```python
from build123d import *

# Parameters (mm, degrees)
F1_DEPTH = 5


with BuildPart() as f1:
    # F0 (on Top) → F1 (new body)
    with BuildSketch(Plane.XY):
        with BuildLine():
            ThreePointArc((-2.891459, -1.483901), (0, 3.25), (2.891459, -1.483901))
            ThreePointArc((2.891459, -1.483901), (2.566364, -2.666148), (2.741421, -3.879717))
            Line((2.741421, -3.879717), (4.605052, -9))
            Line((4.605052, -9), (25, -9))
            Line((25, -9), (25, 2))
            ThreePointArc((25, 2), (23, 4), (25, 6))
            Line((25, 6), (25, 7))
            ThreePointArc((25, 7), (24.707107, 7.707107), (24, 8))
            Line((24, 8), (-24, 8))
            ThreePointArc((-24, 8), (-24.707107, 7.707107), (-25, 7))
            Line((-25, 7), (-25, 6))
            ThreePointArc((-25, 6), (-23, 4), (-25, 2))
            Line((-25, 2), (-25, -9))
            Line((-25, -9), (-4.605052, -9))
            Line((-4.605052, -9), (-2.741421, -3.879717))
            ThreePointArc((-2.741421, -3.879717), (-2.566364, -2.666148), (-2.891459, -1.483901))
        make_face()
    extrude(amount=F1_DEPTH)


solid = f1.part
```
Design review of the part built by this model. Coordinates are the model's own, in mm. A direction names the side the tool comes from. Coordinates: 2 decimals unless noted, no trailing zeros. Order: outer loops, then holes, each group sorted by start corner. A loop starts at its lowest first (then second) coordinate and runs counter-clockwise, first axis right, second up. Notation, with made-up numbers: (60, 14.5) - (75, 14.5) arc R20 cw to (75, 41.5) - close; hole circle Ø6 at (35, -29.75). An arc over 180 degrees is marked (long way). Answer in a Markdown table with one row per item.
(1) Consider section A-A on y = 0. State the section outline as (x, z) points.
Checked values:
| item | result |
|---|---|
| outline | (-25, 0) - (-3.25, 0) - (-3.25, 5) - (-25, 5) - close; (3.25, 0) - (25, 0) - (25, 5) - (3.25, 5) - close |
(2) Consider section C-C on y = 2.5. State the section outline as (x, z) points.
Checked values:
| item | result |
|---|---|
| outline | (-23.68, 0) - (-2.08, 0) - (-2.08, 5) - (-23.68, 5) - close; (2.08, 0) - (23.68, 0) - (23.68, 5) - (2.08, 5) - close |
(3) Consider section B-B on z = 1.4. State the section outline as (x, y) points.
Checked values:
| item | result |
|---|---|
| outline | (-25, -9) - (-4.61, -9) - (-2.74, -3.88) arc R3 ccw to (-2.89, -1.48) arc R3.25 cw (long way) to (2.89, -1.48) arc R3 ccw to (2.74, -3.88) - (4.61, -9) - (25, -9) - (25, 2) arc R2 cw to (25, 6) - (25, 7) arc R1 ccw to (24, 8) - (-24, 8) arc R1 ccw to (-25, 7) - (-25, 6) arc R2 cw to (-25, 2) - close |
(4) Consider section D-D on x = 0. State the section outline as (y, z) points.
Checked values:
| item | result |
|---|---|
| outline | (3.25, 0) - (8, 0) - (8, 5) - (3.25, 5) - close |
(5) The part is to be moulded in two halves that separate along X. For faces 1 (the flat face through (-3.686, -6.476, 2.465)), 2 (the flat face through (-25, -3, 2)), 3 (the flat face through (-0.4, 3.4, 5)), say which applies: released by +X, released by -X, zero draft, split by the parting line, or undercut.
Checked values:
| item | result |
|---|---|
| face 1 | undercut |
| face 2 | released by -X |
| face 3 | zero draft |
(6) For faces 4 (the flat face through (25, -4, 2)), 5 (the flat face through (3.66, -6.4, 2.46)), 6 (the cylindrical face through (2.567, -2.649, 2.465)), list the 3-axis set-ups (+Z, -Z, +X, -X, +Y, -Y) from which the entire face can be reached by the end or side of a thin tool; tool diameter is ignored.
Checked values:
| item | result |
|---|---|
| face 4 | +Z, -Z, +X, +Y, -Y |
| face 5 | +Z, -Z, -Y |
| face 6 | +Z, -Z |
(7) Clearance check with a flat-ended pin moving along its axis: pin 1 (6 mm diameter, centred on x = -9, y = -3, fed in from -Z). State where the tip first meets the part, or that it passes through.
Checked values:
| item | result |
|---|---|
| pin 1 | z = 0 |
(8) Wall thickness on line 1 along X through (y, z) = (0, 1.3); line 2 along X through (y, z) = (-7.75, 0.7); line 3 along Y through (x, z) = (0, 2.8): over which ranges is each line inside the solid? List them lowest first. Write a range as from..to.
Checked values:
| item | result |
|---|---|
| line 1 | -25..-3.25, 3.25..25 |
| line 2 | -25..-4.15, 4.15..25 |
| line 3 | 3.25..8 |
